```python
from build123d import *

# Parameters (mm, degrees)
SKETCH1_W              = 195
SKETCH1_H              = 67
BOSS_EXTRUDE1_DEPTH    = 23
CUT_EXTRUDE1_DEPTH     = 106.629067969
CUT_EXTRUDE2_DEPTH     = 121.516596367
CUT_EXTRUDE3_START     = -13
SKETCH4_W              = 3.612655346
SKETCH4_H              = 3
CUT_EXTRUDE3_DEPTH     = 13
SKETCH6_R              = 2.5
CUT_EXTRUDE4_DEPTH     = 106.629067969
SKETCH7_W              = 37
SKETCH7_H              = 35
CUT_EXTRUDE5_DEPTH     = 1.5
CUT_EXTRUDE6_DEPTH     = 18.5
BOSS_EXTRUDE2_DEPTH    = 55
CUT_EXTRUDE7_OUTLINE_R = 7
CUT_EXTRUDE7_DEPTH     = 81
CUT_EXTRUDE8_START     = -8
SKETCH11_R             = 26
CUT_EXTRUDE8_DEPTH     = 6
SKETCH12_R             = 18.5
CUT_EXTRUDE9_DEPTH     = 167.766303551
SKETCH13_R             = 12.5
CUT_EXTRUDE10_DEPTH    = 54
BOSS_EXTRUDE3_START    = -50
SKETCH14_R             = 18.5
SKETCH14_R_2           = 1.75
SKETCH14_R_3           = 7
BOSS_EXTRUDE3_DEPTH    = 7


# Read off the part's stored shape, not the designer's step: Cut-Extrude7
with BuildPart() as part:
    # Sketch1 → Boss-Extrude1 (new body)
    with BuildSketch(Plane(origin=(0, 0, 0), x_dir=(1, 0, 0), z_dir=(0, 1, 0))):
        Rectangle(SKETCH1_W, SKETCH1_H)
    extrude(amount=BOSS_EXTRUDE1_DEPTH)

    # Sketch2 → Cut-Extrude1 (cut, through all)
    with BuildSketch(Plane.XZ):
        with BuildLine():
            Line((97.5, -3.219751644), (97.5, 33.5))
            Line((97.5, 33.5), (88.5, 33.5))
            ThreePointArc((88.5, 33.5), (95.217186872, 15.683556008), (97.5, -3.219751644))
        make_face()
        with BuildLine():
            Line((97.5, -33.5), (97.5, -3.219751644))
            ThreePointArc((97.5, -3.219751644), (95.985558513, -18.65423771), (91.5, -33.5))
            Line((91.5, -33.5), (97.5, -33.5))
        make_face()
        with BuildLine():
            ThreePointArc((-88, -33.5), (-95.08607052, -15.861694529), (-97.5, 2.992884749))
            Line((-97.5, 2.992884749), (-97.5, -33.5))
            Line((-97.5, -33.5), (-88, -33.5))
        make_face()
        with BuildLine():
            ThreePointArc((-97.5, 2.992884749), (-95.856964648, 18.588830376), (-91, 33.5))
            Line((-91, 33.5), (-97.5, 33.5))
            Line((-97.5, 33.5), (-97.5, 2.992884749))
        make_face()
    extrude(amount=-CUT_EXTRUDE1_DEPTH, mode=Mode.SUBTRACT)

    # Sketch3 → Cut-Extrude2 (cut, through all)
    with BuildSketch(Plane(origin=(0, 0, 33.5), x_dir=(-1, 0, 0), z_dir=(0, 0, -1))):
        Polygon((63.2, 23), (63.2, 12.6), (40.2, 12.6), (40.2, 8.6), (-61.8, 8.6), (-61.8, 12.6), (-97.5, 12.6), (-97.5, 23), align=None)
    extrude(amount=CUT_EXTRUDE2_DEPTH, mode=Mode.SUBTRACT)

    # Sketch4 → Cut-Extrude3 (cut)
    with BuildSketch(Plane(origin=(0, 23, 0), x_dir=(1, 0, 0), z_dir=(0, 1, 0)).offset(CUT_EXTRUDE3_START)):
        with BuildLine():
            Line((-63.2, 30.5), (-63.2, 33.5))
            Line((-63.2, 33.5), (-88, 33.5))
            ThreePointArc((-88, 33.5), (-88.810680862, 32.008999469), (-89.587344654, 30.5))
            Line((-89.587344654, 30.5), (-63.2, 30.5))
        make_face()
        with Locations((-61.393672327, 32)):
            Rectangle(SKETCH4_W, SKETCH4_H)
        with BuildLine():
            Line((-63.2, -33.5), (-63.2, -30.5))
            Line((-63.2, -30.5), (-92.261692194, -30.5))
            ThreePointArc((-92.261692194, -30.5), (-91.647155152, -32.006859002), (-91, -33.5))
            Line((-91, -33.5), (-63.2, -33.5))
        make_face()
        with Locations((-61.393672327, -32)):
            Rectangle(SKETCH4_W, SKETCH4_H)
    extrude(amount=CUT_EXTRUDE3_DEPTH, mode=Mode.SUBTRACT)

    # Sketch6 → Cut-Extrude4 (cut, through all)
    with BuildSketch(Plane.XZ):
        with Locations(Location((-28.1, -9, 0), (0, 0, 270))):
            Circle(SKETCH6_R)
        with Locations(Location((-8.2, -8.3, 0), (0, 0, 270))):
            Circle(SKETCH6_R)
        with Locations(Location((-18.7, 8.7, 0), (0, 0, 270))):
            Circle(SKETCH6_R)
        with Locations(Location((-76.2, 22, 0), (0, 0, 270))):
            Circle(SKETCH6_R)
        with Locations(Location((-78.2, 0.1, 0), (0, 0, 270))):
            Circle(SKETCH6_R)
        with Locations(Location((-73.2, -22.3, 0), (0, 0, 270))):
            Circle(SKETCH6_R)
        with Locations(Location((65.3, -20, 0), (0, 0, 270))):
            Circle(SKETCH6_R)
        with Locations(Location((74.1, -1.7, 0), (0, 0, 270))):
            Circle(SKETCH6_R)
        with Locations(Location((68.3, 21.5, 0), (0, 0, 270))):
            Circle(SKETCH6_R)
    extrude(amount=-CUT_EXTRUDE4_DEPTH, mode=Mode.SUBTRACT)

    # Sketch7 → Cut-Extrude5 (cut)
    with BuildSketch(Plane(origin=(0, 8.6, 0), x_dir=(1, 0, 0), z_dir=(0, 1, 0))):
        with Locations((5.3, -16)):
            Rectangle(SKETCH7_W, SKETCH7_H)
    extrude(amount=-CUT_EXTRUDE5_DEPTH, mode=Mode.SUBTRACT)

    # Sketch8 → Cut-Extrude6 (cut)
    with BuildSketch(Plane(origin=(0, 23, 0), x_dir=(1, 0, 0), z_dir=(0, 1, 0))):
        with BuildLine():
            Line((37.096152423, 33.5), (31.9, 33.5))
            Line((31.9, 33.5), (31.9, 30.5))
            ThreePointArc((31.9, 30.5), (34.9, 31.303847577), (37.096152423, 33.5))
        make_face()
        with BuildLine():
            Line((31.9, 33.5), (26.703847577, 33.5))
            ThreePointArc((26.703847577, 33.5), (28.9, 31.303847577), (31.9, 30.5))
            Line((31.9, 30.5), (31.9, 33.5))
        make_face()
    extrude(amount=-CUT_EXTRUDE6_DEPTH, mode=Mode.SUBTRACT)

    # Sketch9 → Boss-Extrude2 (add)
    with BuildSketch(Plane.XZ):
        Polygon((-83.5, -27), (-83.5, -40.5), (135, -40.5), (135, 40.5), (-83.5, 40.5), (-83.5, 27), (81.5, 27), (81.5, 0), (81.5, -27), align=None)
    extrude(amount=BOSS_EXTRUDE2_DEPTH)

    # Cut-Extrude7 outline → Cut-Extrude7 (cut)
    with BuildSketch(Plane(origin=(-0.000736395, 0, 40.5), x_dir=(-1, 0, 0), z_dir=(0, 0, -1))):
        with BuildLine():
            Line((83.499263605, -55), (83.499263605, 0))
            ThreePointArc((83.499263605, 0), (79.744905458, -4.369344862), (74.219749945, -6))
            Line((74.219749945, -6), (40.329566384, -6))
            ThreePointArc((40.329566384, -6), (31.649853034, -31.517594688), (5.442617021, -25.219512195))
            ThreePointArc((5.442617021, -25.219512195), (-9.896457675, -16.099848766), (-26.712562231, -22.072628782))
            Line((-26.712562231, -22.072628782), (-51.806469277, -46.903161625))
            ThreePointArc((-51.806469277, -46.903161625), (-60.853871258, -52.896800241), (-71.500736395, -55))
            Line((-71.500736395, -55), (83.499263605, -55))
        make_face()
        Polygon((87.999263605, 10), (83.499263605, 0), (97.499263605, 0), (97.499263605, 23), (87.999263605, 23), align=None)
        with Locations((-71.500736395, -27)):
            Circle(CUT_EXTRUDE7_OUTLINE_R)
        with Locations((21.999263605, -14)):
            Circle(CUT_EXTRUDE7_OUTLINE_R)
    extrude(amount=CUT_EXTRUDE7_DEPTH, mode=Mode.SUBTRACT)

    # Sketch11 → Cut-Extrude8 (cut)
    with BuildSketch(Plane.XY.offset(CUT_EXTRUDE8_START)):
        with Locations((71.5, -27)):
            Circle(SKETCH11_R)
    extrude(amount=-CUT_EXTRUDE8_DEPTH, mode=Mode.SUBTRACT)

    # Sketch12 → Cut-Extrude9 (cut, through all)
    with BuildSketch(Plane.XY.offset(40.5)):
        with Locations((108.5, -27)):
            Circle(SKETCH12_R)
    extrude(amount=-CUT_EXTRUDE9_DEPTH, mode=Mode.SUBTRACT)

    # Sketch13 → Cut-Extrude10 (cut)
    with BuildSketch(Plane.XY.offset(-27)):
        with Locations((71.5, -27)):
            Circle(SKETCH13_R)
    extrude(amount=CUT_EXTRUDE10_DEPTH, mode=Mode.SUBTRACT)

    # Sketch14 → Boss-Extrude3 (add)
    with BuildSketch(Plane(origin=(0, 0, -40.5), x_dir=(-1, 0, 0), z_dir=(0, 0, -1)).offset(BOSS_EXTRUDE3_START)):
        with Locations(Location((-108.5, -27, 0), (0, 0, 180))):
            Circle(SKETCH14_R)
        with Locations((-108.5, -11.5)):
            Circle(SKETCH14_R_2, mode=Mode.SUBTRACT)
        with Locations((-95.076606241, -19.25)):
            Circle(SKETCH14_R_2, mode=Mode.SUBTRACT)
        with Locations((-95.076606241, -34.75)):
            Circle(SKETCH14_R_2, mode=Mode.SUBTRACT)
        with Locations((-108.5, -42.5)):
            Circle(SKETCH14_R_2, mode=Mode.SUBTRACT)
        with Locations((-121.923393759, -34.75)):
            Circle(SKETCH14_R_2, mode=Mode.SUBTRACT)
        with Locations((-121.923393759, -19.25)):
            Circle(SKETCH14_R_2, mode=Mode.SUBTRACT)
        with Locations((-101.5, -27)):
            Circle(SKETCH14_R_3, mode=Mode.SUBTRACT)
    extrude(amount=BOSS_EXTRUDE3_DEPTH)


solid = part.part
```
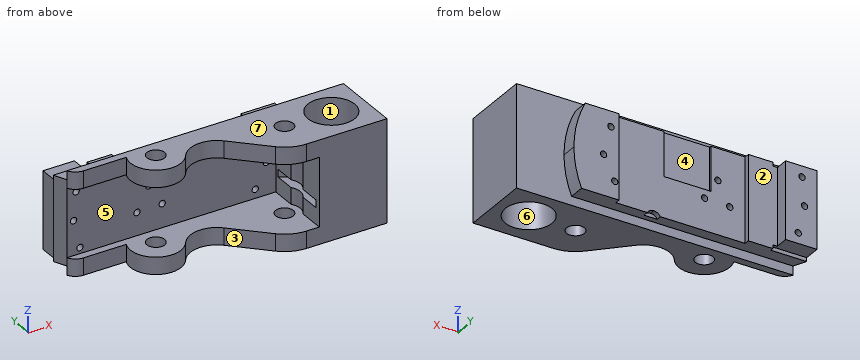
Input: part model. Units: mm. Frame: model coordinates. Face numbers are marked on the shaded views. A direction names the side the tool comes from. Give positions to 0.01 mm unless a question says otherwise; leave off trailing zeros. Loops run counter-clockwise (first coordinate to the right, second up) from the corner with the lowest first, then second, coordinate; pieces in that order, holes last.
1) Section query B-B on x = 74.1. Return the cut outline in (y, z), and give its area (3 significant figures).
A:
outline: (-55, -40.5) - (-33.5, -40.5) - (-33.5, -27) - (-55, -27) - close; (-55, 27) - (-33.5, 27) - (-33.5, 40.5) - (-55, 40.5) - close; (-20.5, -40.5) - (0, -40.5) - (0, -33.5) - (12.6, -33.5) - (12.6, -4.2) - (0, -4.2) - (0, -27) - (-20.5, -27) - close; (-20.5, 27) - (0, 27) - (0, 0.8) - (12.6, 0.8) - (12.6, 33.5) - (0, 33.5) - (0, 40.5) - (-20.5, 40.5) - close
area: 1,920 mm2
2) Section query C-C on x = -8.2. Return the cut outline in (y, z), and give its area (3 significant figures).
A:
outline: (-28.48, -40.5) - (0, -40.5) - (0, -33.5) - (8.6, -33.5) - (8.6, -10.8) - (0, -10.8) - (0, -27) - (-28.48, -27) - close; (-28.48, 27) - (0, 27) - (0, -5.8) - (8.6, -5.8) - (8.6, -1.5) - (7.1, -1.5) - (7.1, 33.5) - (0, 33.5) - (0, 40.5) - (-28.48, 40.5) - close
area: 1,250 mm2
3) Mould query, pull axis Y, two halves, no side actions, for the marked faces 5, 6 and 7. Classes: released by +Y, released by -Y, zero draft, split by the parting line, or undercut.
A:
face 5: released by -Y
face 6: undercut
face 7: zero draft
4) Section query D-D on x = 21. Return the cut outline in (y, z), and give its area (3 significant figures).
A:
outline: (-18.05, -40.5) - (0, -40.5) - (0, -33.5) - (8.6, -33.5) - (8.6, -1.5) - (7.1, -1.5) - (7.1, 33.5) - (0, 33.5) - (0, 40.5) - (-18.05, 40.5) - (-18.05, 27) - (0, 27) - (0, -27) - (-18.05, -27) - close
area: 1,010 mm2
5) Reachability of the marked faces 1, 2, 3 and 4 from +Z, -Z, +X, -X, +Y, -Y: full face, straight path, thin tool, end or side. Return the list, or none.
A:
face 1: +Z
face 2: +Z, -Z, +X, +Y
face 3: +Z, -Z, -Y
face 4: +Z, +Y
6) Contact query for flat-ended pins moving along their axis: pin 1 (6.5 mm diameter, centred on x = 68.3, z = 21.5, fed in from -Y); pin 2 (2 mm diameter, centred on x = 108.5, y = -42.5, fed in from -Z); pin 3 (6 mm diameter, centred on x = -56.5, z = 29.5, fed in from +Y); pin 4 (22.5 mm diameter, centred on y = -45, z = -11.5, fed in from -X). Output: stop coordinate, or through.
A:
pin 1: stops at y = 0
pin 2: passes through
pin 3: stops at y = 12.6
pin 4: stops at x = 81.5
7) Line query: L1, parallel to Z at x = -8, y = 4; L2, parallel to Z at x = -32.5, y = -10; L3, parallel to X at y = -14, z = 36. Output: solid intervals per line, ascending.
A:
L1: z = -33.5 to -10.79, -5.81 to 33.5
L2: z = -40.5 to -27, 27 to 40.5
L3: x = -42 to -29, -15 to 95.34, 121.66 to 135
8) Section query A-A on z = 21.5. Count the separate pieces of the cut face and the enclosed holes in it, and give its area (3 significant figures).
A:
separate pieces: 3
enclosed holes: 1
area: 3,730 mm2
